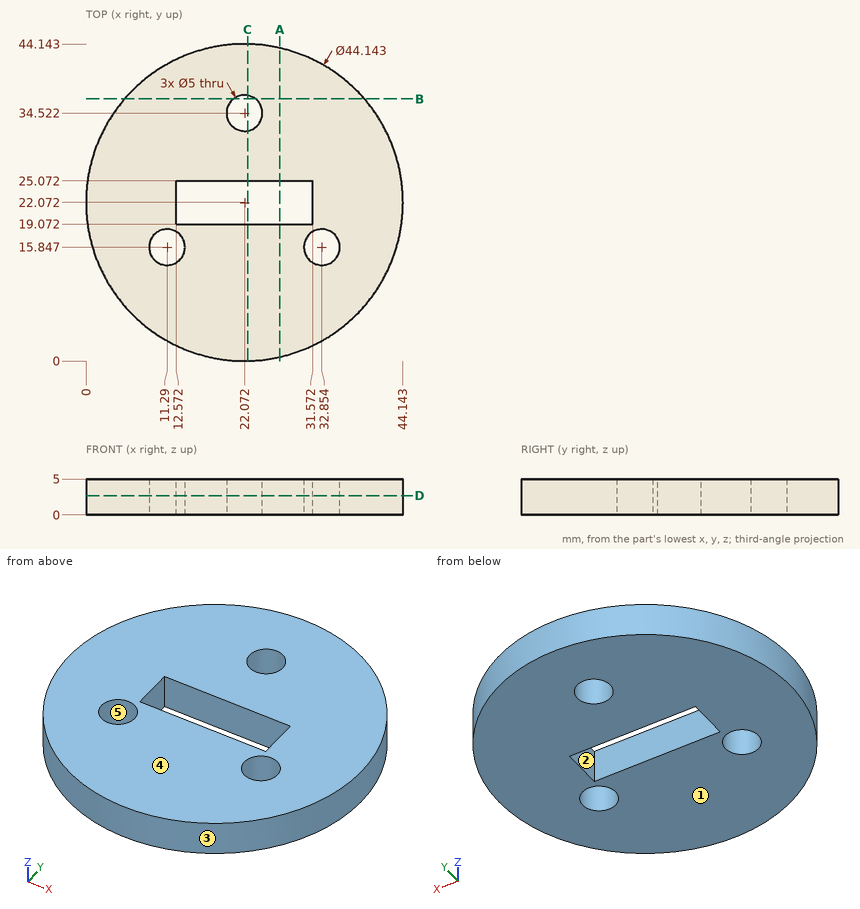
Check sheet for the drawn part. Datum: minimum x, y, z corner. Units: mm. A direction names the side the tool comes from. Give positions to 0.01 mm unless a question says otherwise; leave off trailing zeros. Loops run counter-clockwise (first coordinate to the right, second up) from the corner with the lowest first, then second, coordinate; pieces in that order, holes last. Notation, with made-up numbers: M -28,-20.75 L -14,-20.75 A29 ccw -14,14.25 Z; hole C -31.75,71 d10. An arc over 180 degrees is marked long. Return JSON: item names as keys, results as strings.
1) Section check D-D, the plane z = 2.7. Enter the section's corners in (x, y), and give its area (3 significant figures).
Findings:
{"outline": "C 22.07,22.07 d44.14; hole C 11.29,15.85 d5; hole M 12.57,19.07 L 31.57,19.07 L 31.57,25.07 L 12.57,25.07 Z; hole C 22.07,34.52 d5; hole C 32.85,15.85 d5", "area": "1,360 mm2"}
2) Mould release check, pull along Y, two halves, no side actions. Record for the marked faces 3, 4 and 5: released by +Y, released by -Y, zero draft, split by the parting line, or undercut.
Findings:
{"face 3": "split by the parting line", "face 4": "zero draft", "face 5": "undercut"}
3) Section check A-A, the plane x = 27. Enter the section's corners in (y, z), and give its area (3 significant figures).
Findings:
{"outline": "M 0.56,0 L 19.07,0 L 19.07,5 L 0.56,5 Z; M 25.07,0 L 43.59,0 L 43.59,5 L 25.07,5 Z", "area": "185 mm2"}
4) Section check B-B, the plane y = 36.5. Enter the section's corners in (x, z) (1 decimal), and give its area (3 significant figures).
Findings:
{"outline": "M 5.4,0 L 20.5,0 L 20.5,5 L 5.4,5 Z; M 23.6,0 L 38.8,0 L 38.8,5 L 23.6,5 Z", "area": "152 mm2"}
5) Material ranges on L1, parallel to X at y = 18, z = 0.6 (1 decimal); L2, parallel to X at y = 22.5, z = 3.75; L3, parallel to Y at x = 21.5, z = 0.35 (1 decimal), recorded low to high. Write a range as [from, to].
Findings:
{"L1": "x = [0.4, 10], [12.6, 31.6], [34.1, 43.8]", "L2": "x = [0, 12.57], [31.57, 44.14]", "L3": "y = [0, 19.1], [25.1, 32.1], [37, 44.1]"}
6) Tool access check on the marked faces 1 and 2. Record the directions out of +Z, -Z, +X, -X, +Y, -Y that give a thin tool (end or side, any length) a straight path to the whole face; none if there is none.
Findings:
{"face 1": "-Z, +X, -X, +Y, -Y", "face 2": "+Z, -Z"}
7) Gauge pin test, flat ends, axial feed: P1, Ø3, axis at x = 11.29, y = 15.85, coming from the +Z side; P2, Ø1.5, axis at x = 12, z = 2, coming from the -Y side (1 decimal); P3, Ø2, axis at x = 22, z = 4.5, coming from the -Y side; P4, Ø1.5, axis at y = 23, z = 3.5, coming from the -X side. Record the tip position at first contact, or that the pin passes through.
Findings:
{"P1": "passes through", "P2": "stops at y = 2.1", "P3": "stops at y = 0", "P4": "stops at x = 0"}
8) Section check C-C, the plane x = 22.5. Enter the section's corners in (y, z) (1 decimal), and give its area (3 significant figures).
Findings:
{"outline": "M 0,0 L 19.1,0 L 19.1,5 L 0,5 Z; M 25.1,0 L 32.1,0 L 32.1,5 L 25.1,5 Z; M 37,0 L 44.1,0 L 44.1,5 L 37,5 Z", "area": "166 mm2"}
